```python
from build123d import *

# Parameters (mm, degrees)
SKETCH_W        = 89.16
SKETCH_H        = 54.87
PAD_DEPTH       = 6
POCKET_DEPTH    = 4.6
SKETCH002_W     = 86.56
SKETCH002_H     = 52.27
POCKET001_DEPTH = 1.6
SKETCH004_R     = 1.2
POCKET002_DEPTH = 2.2
SKETCH003_R     = 2.1
POCKET003_DEPTH = 2
SKETCH005_W     = 44.45
SKETCH005_H     = 4
PAD001_DEPTH    = 2
CHAMFER_SIZE    = 1


with BuildPart() as part:
    # Sketch → Pad (new body)
    with BuildSketch(Plane.XY):
        with Locations((44.58, 27.435)):
            Rectangle(SKETCH_W, SKETCH_H)
    extrude(amount=PAD_DEPTH)

    # Sketch001 → Pocket (cut)
    with BuildSketch(Plane.XY.offset(6)):
        with BuildLine():
            ThreePointArc((3.94, 46.93), (6.768427, 48.101573), (7.94, 50.93))
            Line((7.94, 50.93), (7.94, 53.47))
            Line((7.94, 53.47), (36.77, 53.47))
            Line((36.77, 53.47), (36.77, 50.93))
            ThreePointArc((36.77, 50.93), (40.77, 46.93), (44.77, 50.93))
            Line((44.77, 50.93), (44.77, 53.47))
            Line((44.77, 53.47), (81.22, 53.47))
            Line((81.22, 53.47), (81.22, 50.93))
            ThreePointArc((81.22, 50.93), (82.391573, 48.101573), (85.22, 46.93))
            Line((85.22, 46.93), (87.76, 46.93))
            Line((87.76, 46.93), (87.76, 7.94))
            Line((87.76, 7.94), (85.22, 7.94))
            ThreePointArc((85.22, 7.94), (82.391573, 6.768427), (81.22, 3.94))
            Line((81.22, 1.4), (81.22, 3.94))
            Line((44.77, 1.4), (81.22, 1.4))
            Line((44.77, 3.94), (44.77, 1.4))
            ThreePointArc((44.77, 3.94), (40.77, 7.94), (36.77, 3.94))
            Line((36.77, 1.4), (36.77, 3.94))
            Line((7.94, 1.4), (36.77, 1.4))
            Line((7.94, 3.94), (7.94, 1.4))
            ThreePointArc((7.94, 3.94), (6.768427, 6.768427), (3.94, 7.94))
            Line((1.4, 7.94), (3.94, 7.94))
            Line((1.4, 46.93), (1.4, 7.94))
            Line((3.94, 46.93), (1.4, 46.93))
        make_face()
    extrude(amount=-POCKET_DEPTH, mode=Mode.SUBTRACT)

    # Sketch002 → Pocket001 (cut)
    with BuildSketch(Plane.XY.offset(6)):
        with Locations((44.58, 27.435)):
            Rectangle(SKETCH002_W, SKETCH002_H)
    extrude(amount=-POCKET001_DEPTH, mode=Mode.SUBTRACT)

    # Sketch004 → Pocket002 (cut)
    with BuildSketch(Plane.XY.offset(4.4)):
        with Locations((3.94, 50.93)):
            Circle(SKETCH004_R)
        with Locations((40.77, 50.93)):
            Circle(SKETCH004_R)
        with Locations((85.22, 50.93)):
            Circle(SKETCH004_R)
        with Locations((85.22, 3.94)):
            Circle(SKETCH004_R)
        with Locations((40.77, 3.94)):
            Circle(SKETCH004_R)
        with Locations((3.94, 3.94)):
            Circle(SKETCH004_R)
    extrude(amount=-POCKET002_DEPTH, mode=Mode.SUBTRACT)

    # Sketch003 → Pocket003 (cut)
    with BuildSketch(Plane(origin=(0, 0, 0), x_dir=(1, 0, 0), z_dir=(0, 0, -1))):
        with Locations((3.94, -3.94)):
            Circle(SKETCH003_R)
        with Locations((40.77, -3.94)):
            Circle(SKETCH003_R)
        with Locations((85.22, -3.94)):
            Circle(SKETCH003_R)
        with Locations((85.22, -50.93)):
            Circle(SKETCH003_R)
        with Locations((40.77, -50.93)):
            Circle(SKETCH003_R)
        with Locations((3.94, -50.93)):
            Circle(SKETCH003_R)
    extrude(amount=-POCKET003_DEPTH, mode=Mode.SUBTRACT)

    # Sketch005 → Pad001 (new body)
    with BuildSketch(Plane.XY.offset(1.4)):
        with Locations((62.995, 27.435)):
            Rectangle(SKETCH005_W, SKETCH005_H)
    extrude(amount=PAD001_DEPTH)

    # Chamfer
    chamfer_edges = [part.edges().sort_by_distance(p)[0] for p in [
        (44.58, 54.87, 0),
        (89.16, 27.435, 0),
        (0, 27.435, 0),
        (44.58, 0, 0),
    ]]
    chamfer(chamfer_edges, length=CHAMFER_SIZE)


solid = part.part
```
Model file for the job. Use its own axes, mm. A direction names the side the tool comes from. Give positions to 0.01 mm unless a question says otherwise; leave off trailing zeros. Loops run counter-clockwise (first coordinate to the right, second up) from the corner with the lowest first, then second, coordinate; pieces in that order, holes last. Notation, with made-up numbers: (54.5, 39) -> (71.5, 39) arc R22 ccw to (71.5, 47) -> close; hole circle Ø4 at (49, -39.5). An arc over 180 degrees is marked (long way). Write each question's results on one line, items separated by ' | '.
(1) Cut at B-B on x = 21.5. List the corners of the cut face in (y, z), and give its area (3 significant figures).
Geometry results:
outline: (0, 1) -> (1, 0) -> (53.87, 0) -> (54.87, 1) -> (54.87, 6) -> (53.57, 6) -> (53.57, 4.4) -> (53.47, 4.4) -> (53.47, 1.4) -> (1.4, 1.4) -> (1.4, 4.4) -> (1.3, 4.4) -> (1.3, 6) -> (0, 6) -> close | area: 88.4 mm²
(2) Pull direction X, two halves, no side cores. Call faces 1 (the flat face through (44, 28, 0)), 2 (the flat face through (40.77, 27, 2)): released by +X, released by -X, zero draft, split by the parting line, or undercut.
Geometry results:
face 1: zero draft | face 2: undercut
(3) Probe line 1 along Y through (x, z) = (62, 2.7) (3 decimals); line 2 along X through (y, z) = (14.5, 4.7); line 3 along Y through (x, z) = (73.5, 3.5). List the from-to ranges inside material, lowest first.
Geometry results:
line 1: y = 0 to 1.4, 25.435 to 29.435, 53.47 to 54.87 | line 2: x = 0 to 1.3, 87.86 to 89.16 | line 3: y = 0 to 1.4, 53.47 to 54.87
(4) Cut at A-A on y = 28. List the corners of the cut face in (x, z), and give its area (3 significant figures).
Geometry results:
outline: (0, 1) -> (1, 0) -> (88.16, 0) -> (89.16, 1) -> (89.16, 6) -> (87.86, 6) -> (87.86, 4.4) -> (87.76, 4.4) -> (87.76, 1.4) -> (85.22, 1.4) -> (85.22, 3.4) -> (40.77, 3.4) -> (40.77, 1.4) -> (1.4, 1.4) -> (1.4, 4.4) -> (1.3, 4.4) -> (1.3, 6) -> (0, 6) -> close | area: 225 mm²
(5) Cut at C-C on x = 80. List the corners of the cut face in (y, z) (3 decimals), and give its area (3 significant figures).
Geometry results:
outline: (0, 1) -> (1, 0) -> (53.87, 0) -> (54.87, 1) -> (54.87, 6) -> (53.57, 6) -> (53.57, 4.4) -> (53.47, 4.4) -> (53.47, 1.4) -> (29.435, 1.4) -> (29.435, 3.4) -> (25.435, 3.4) -> (25.435, 1.4) -> (1.4, 1.4) -> (1.4, 4.4) -> (1.3, 4.4) -> (1.3, 6) -> (0, 6) -> close | area: 96.4 mm²
(6) Tool access for faces 3 (the flat face through (41, 4, 2.2)), 4 (the flat face through (44, 54.87, 3)), 5 (the cylindrical face through (41.9, 49.16, 0.99)): list every direction of +Z, -Z, +X, -X, +Y, -Y with a clear straight run to the whole face (end or side of a thin tool).
Geometry results:
face 3: +Z | face 4: +Z, -Z, +X, -X, +Y | face 5: -Z
(7) Flat gauge pins, fed straight in: pin 1 Ø2.5 at (x, y) = (3.94, 50.93) entering from -Z; pin 2 Ø0.7 at (x, y) = (3.5, 51) entering from +Z; pin 3 Ø5 at (x, y) = (23, 48.5) entering from +Z. Where does each tip first touch, or does it go through?
Geometry results:
pin 1: stops at z = 2 | pin 2: stops at z = 2.2 | pin 3: stops at z = 1.4
